```python
from build123d import *

# Parameters (mm, degrees)
SKETCH_1_W          = 140
SKETCH_1_H          = 220
SKETCH_1_R          = 1.75
SKETCH_1_R_2        = 20
EXTRUDE_1_DEPTH     = 3
SKETCH_2_R          = 1.75
SKETCH_2_R_2        = 2
SKETCH_2_R_3        = 5
CUT_EXTRUDE_1_DEPTH = 131.418556962
SKETCH_3_R          = 1.75
CUT_EXTRUDE_2_DEPTH = 131.418556962
CUT_EXTRUDE_3_DEPTH = 131.418556962


with BuildPart() as part:
    # 草图1 → 凸台-拉伸1 (new body)
    with BuildSketch(Plane(origin=(0, 0, 0), x_dir=(1, 0, 0), z_dir=(0, 1, 0))):
        Rectangle(SKETCH_1_W, SKETCH_1_H)
        with Locations(Location((-5.8, -59, 0), (0, 0, 270))):
            Circle(SKETCH_1_R, mode=Mode.SUBTRACT)
        with Locations(Location((25.7, -59, 0), (0, 0, 270))):
            Circle(SKETCH_1_R, mode=Mode.SUBTRACT)
        with Locations(Location((-5.8, -107, 0), (0, 0, 270))):
            Circle(SKETCH_1_R, mode=Mode.SUBTRACT)
        with Locations(Location((25.7, -107, 0), (0, 0, 270))):
            Circle(SKETCH_1_R, mode=Mode.SUBTRACT)
        with Locations(Location((0, -32, 0), (0, 0, 270))):
            Circle(SKETCH_1_R_2, mode=Mode.SUBTRACT)
    extrude(amount=EXTRUDE_1_DEPTH)

    # 草图2 → 切除-拉伸1 (cut, through all)
    with BuildSketch(Plane(origin=(0, 3, 0), x_dir=(1, 0, 0), z_dir=(0, 1, 0))):
        with Locations(Location((48, -62, 0), (0, 0, 270))):
            Circle(SKETCH_2_R)
        with Locations(Location((62, -62, 0), (0, 0, 270))):
            Circle(SKETCH_2_R)
        with Locations(Location((62, -78, 0), (0, 0, 270))):
            Circle(SKETCH_2_R)
        with Locations(Location((48, -78, 0), (0, 0, 270))):
            Circle(SKETCH_2_R)
        with Locations(Location((-62, -78, 0), (0, 0, 90))):
            Circle(SKETCH_2_R)
        with Locations(Location((-48, -78, 0), (0, 0, 90))):
            Circle(SKETCH_2_R)
        with Locations(Location((-62, -62, 0), (0, 0, 90))):
            Circle(SKETCH_2_R)
        with Locations(Location((-48, -62, 0), (0, 0, 90))):
            Circle(SKETCH_2_R)
        with Locations(Location((-35, 70, 0), (0, 0, 270))):
            Circle(SKETCH_2_R)
        with Locations(Location((-35, -70, 0), (0, 0, 270))):
            Circle(SKETCH_2_R)
        with Locations(Location((35, -70, 0), (0, 0, 270))):
            Circle(SKETCH_2_R)
        with Locations(Location((35, 70, 0), (0, 0, 270))):
            Circle(SKETCH_2_R)
        with Locations(Location((-20, 70, 0), (0, 0, 270))):
            Circle(SKETCH_2_R_2)
        with Locations(Location((20, 70, 0), (0, 0, 270))):
            Circle(SKETCH_2_R_2)
        with Locations(Location((55, -70, 0), (0, 0, 270))):
            Circle(SKETCH_2_R_3)
        with Locations(Location((-55, -70, 0), (0, 0, 90))):
            Circle(SKETCH_2_R_3)
    extrude(amount=-CUT_EXTRUDE_1_DEPTH, mode=Mode.SUBTRACT)

    # 草图3 → 切除-拉伸2 (cut, through all)
    with BuildSketch(Plane(origin=(0, 3, 0), x_dir=(1, 0, 0), z_dir=(0, 1, 0))):
        with Locations(Location((55, -90, 0), (0, 0, 270))):
            Circle(SKETCH_3_R)
        with Locations(Location((-55, -90, 0), (0, 0, 270))):
            Circle(SKETCH_3_R)
        with Locations(Location((64.5, -47.5, 0), (0, 0, 270))):
            Circle(SKETCH_3_R)
        with Locations(Location((27.5, -47.5, 0), (0, 0, 270))):
            Circle(SKETCH_3_R)
        with Locations(Location((64.5, 13.5, 0), (0, 0, 270))):
            Circle(SKETCH_3_R)
        with Locations(Location((27.5, 13.5, 0), (0, 0, 270))):
            Circle(SKETCH_3_R)
        with Locations(Location((-25.25, -52.75, 0), (0, 0, 270))):
            Circle(SKETCH_3_R)
        with Locations(Location((-61.75, -16.25, 0), (0, 0, 270))):
            Circle(SKETCH_3_R)
        with Locations(Location((-25.25, -16.25, 0), (0, 0, 270))):
            Circle(SKETCH_3_R)
        with Locations(Location((-60, -6, 0), (0, 0, 270))):
            Circle(SKETCH_3_R)
        with Locations(Location((24, 62, 0), (0, 0, 270))):
            Circle(SKETCH_3_R)
        with Locations(Location((-60, 62, 0), (0, 0, 270))):
            Circle(SKETCH_3_R)
        with Locations(Location((-61.75, -52.75, 0), (0, 0, 270))):
            Circle(SKETCH_3_R)
    extrude(amount=-CUT_EXTRUDE_2_DEPTH, mode=Mode.SUBTRACT)

    # 草图5 → 切除-拉伸3 (cut, through all)
    with BuildSketch(Plane(origin=(0, 3, 0), x_dir=(1, 0, 0), z_dir=(0, 1, 0))):
        with BuildLine():
            Line((-35, 80), (35, 80))
            ThreePointArc((35, 80), (59.748737342, 69.748737342), (70, 45))
            Line((70, 45), (70, 110))
            Line((70, 110), (-70, 110))
            Line((-70, 110), (-70, 45))
            ThreePointArc((-70, 45), (-59.748737342, 69.748737342), (-35, 80))
        make_face()
    extrude(amount=-CUT_EXTRUDE_3_DEPTH, mode=Mode.SUBTRACT)


solid = part.part
```
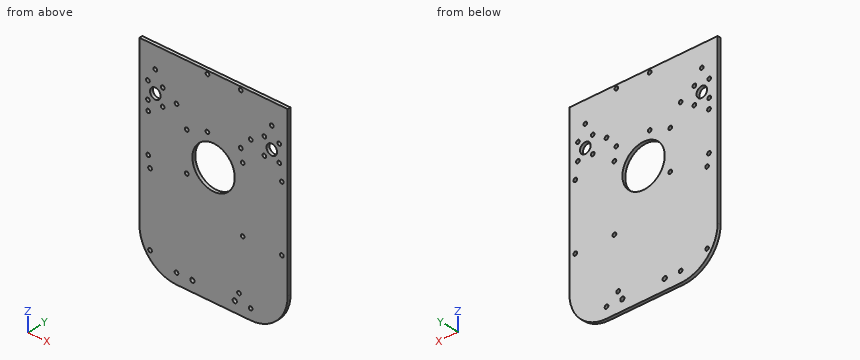
Can you work these out from the model? Positions are in its coordinate system, mm. Coordinates: 2 decimals unless noted, no trailing zeros. Loops run counter-clockwise (first coordinate to the right, second up) from the corner with the lowest first, then second, coordinate; pieces in that order, holes last. Notation, with made-up numbers: (-10, -26.75) - (26, -26.75) arc R21 ccw to (26, 4.25) - close; hole circle Ø3 at (68.25, -28). An arc over 180 degrees is marked (long way). Answer as CSV lines item,"result". Start each with the question number.
1) I need wall thicknesses on line 1 (X direction, y = 2.35, z = 70); line 2 (Z direction, x = -54.5, y = 0.2); line 3 (Z direction, x = 25, y = 0.25). Which ranges of each line are inside material? Lowest first, please. Write a range as from..to.
2) Suppose I cut it at B-B (y = 0.5). Count the separate pieces of the cut face and the enclosed holes in it, plus the area to 3 significant figures.
3) Suppose I cut it at A-A (z = 20). Please give me the cut outline in (x, y), plus the area to 3 significant figures.
Check result:
1,line 1,"x = -70..-60, -50..-36.75, -33.25..33.25, 36.75..50, 60..70"
1,line 2,"z = -74.06..65.03, 74.97..88.32, 91.68..110"
1,line 3,"z = -80..-63.44, -60.56..57.4, 60.6..105.4, 108.6..110"
2,separate pieces,"1"
2,enclosed holes,"34"
2,area,"24,400 mm²"
3,outline,"(-70, 0) - (-16, 0) - (-16, 3) - (-70, 3) - close; (16, 0) - (70, 0) - (70, 3) - (16, 3) - close"
3,area,"324 mm²"
